```python
from build123d import *

# Parameters (mm, degrees)
SKETCH_1_W                  = 60
SKETCH_1_H                  = 100
EXTRUDE_1_DEPTH             = 2.9718
SKETCH_2_W                  = 2.9718
SKETCH_2_H                  = 40
CUT_EXTRUDE_1_DEPTH         = 10
SKETCH_4_W                  = 60
SKETCH_4_H                  = 30
EXTRUDE_2_DEPTH             = 2.9718
CUT_EXTRUDE_2_DEPTH         = 2.9718
PATTERN_LINEAR_1_COUNT      = 3
PATTERN_LINEAR_1_PITCH      = 8
SKETCH_5_R                  = 1
CUT_EXTRUDE_3_DEPTH         = 10
PATTERN_LINEAR_2_COUNT      = 3
PATTERN_LINEAR_2_PITCH      = 8
PATTERN_LINEAR_2_COUNT_DIR2 = 2
PATTERN_LINEAR_2_PITCH_DIR2 = 30
CUT_EXTRUDE_4_DEPTH         = 10
SKETCH_8_R                  = 1.4
CUT_EXTRUDE_5_DEPTH         = 10
PATTERN_LINEAR_3_COUNT      = 4
PATTERN_LINEAR_3_PITCH      = 70


with BuildPart() as part:
    # 草图1 → 凸台-拉伸1 (new body)
    with BuildSketch(Plane(origin=(0, 0, 0), x_dir=(1, 0, 0), z_dir=(0, 1, 0))):
        Rectangle(SKETCH_1_W, SKETCH_1_H)
    extrude(amount=EXTRUDE_1_DEPTH)

    # 草图2 → 切除-拉伸1 (cut)
    with BuildSketch(Plane(origin=(0, 0, 0), x_dir=(-1, 0, 0), z_dir=(0, -1, 0))):
        with Locations((28.5141, 0)):
            Rectangle(SKETCH_2_W, SKETCH_2_H)
    extrude(amount=-CUT_EXTRUDE_1_DEPTH, mode=Mode.SUBTRACT)

    # 草图4 → 凸台-拉伸2 (add)
    with BuildSketch(Plane.XZ):
        with Locations((0, -65)):
            Rectangle(SKETCH_4_W, SKETCH_4_H)
    extrude(amount=-EXTRUDE_2_DEPTH)

    # 草图3 → 切除-拉伸2 (cut)
    with BuildSketch(Plane(origin=(0, 0, 0), x_dir=(-1, 0, 0), z_dir=(0, -1, 0))):
        with BuildLine():
            Line((-12.5, 55.002516758), (-30, 55.002516758))
            Line((-30, 55.002516758), (-30, 53.002516758))
            Line((-30, 53.002516758), (-12.5, 53.002516758))
            ThreePointArc((-12.5, 53.002516758), (-11.5, 54.002516758), (-12.5, 55.002516758))
        make_face()
        with BuildLine():
            Line((30, 53.002516758), (30, 55.002516758))
            Line((30, 55.002516758), (12.5, 55.002516758))
            ThreePointArc((12.5, 55.002516758), (11.5, 54.002516758), (12.5, 53.002516758))
            Line((12.5, 53.002516758), (30, 53.002516758))
        make_face()
        with BuildLine():
            Line((8, 55.002516758), (-8, 55.002516758))
            ThreePointArc((-8, 55.002516758), (-9, 54.002516758), (-8, 53.002516758))
            Line((-8, 53.002516758), (8, 53.002516758))
            ThreePointArc((8, 53.002516758), (9, 54.002516758), (8, 55.002516758))
        make_face()
    cut_extrude_2 = extrude(amount=-CUT_EXTRUDE_2_DEPTH, mode=Mode.SUBTRACT)

    # 阵列(线性)1: 切除-拉伸2 ×3
    with Locations(*[(0, 0, -i * PATTERN_LINEAR_1_PITCH) for i in range(1, PATTERN_LINEAR_1_COUNT)]):
        add(cut_extrude_2, mode=Mode.SUBTRACT)

    # 草图5 → 切除-拉伸3 (cut)
    with BuildSketch(Plane.XZ):
        with BuildLine():
            Line((-5, -57.002516758), (-25, -57.002516758))
            ThreePointArc((-25, -57.002516758), (-24.292893219, -57.295409977), (-24, -58.002516758))
            ThreePointArc((-24, -58.002516758), (-24.292893219, -58.709623539), (-25, -59.002516758))
            Line((-25, -59.002516758), (-5, -59.002516758))
            ThreePointArc((-5, -59.002516758), (-6, -58.002516758), (-5, -57.002516758))
        make_face()
        with Locations((-25, -58.002516758)):
            Circle(SKETCH_5_R)
        with Locations((-5, -58.002516758)):
            Circle(SKETCH_5_R)
    cut_extrude_3 = extrude(amount=-CUT_EXTRUDE_3_DEPTH, mode=Mode.SUBTRACT)

    # 阵列(线性)2: Cut-Extrude 3 3 × 2
    with Locations(*[(j * PATTERN_LINEAR_2_PITCH_DIR2, 0, -i * PATTERN_LINEAR_2_PITCH) for i in range(PATTERN_LINEAR_2_COUNT) for j in range(PATTERN_LINEAR_2_COUNT_DIR2) if (i, j) != (0, 0)]):
        add(cut_extrude_3, mode=Mode.SUBTRACT)

    # 草图7 → 切除-拉伸4 (cut)
    with BuildSketch(Plane.XZ):
        Polygon((-30, 1.5), (-30, 0), (-15, 0), (-15, 1.5), (-19.5, 1.5), (-19.5, 4), (-22, 4), (-22, 1.5), align=None)
        Polygon((-30, 0), (-30, -1.5), (-22, -1.5), (-22, -4), (-19.5, -4), (-19.5, -1.5), (-15, -1.5), (-15, 0), align=None)
    extrude(amount=-CUT_EXTRUDE_4_DEPTH, mode=Mode.SUBTRACT)

    # 草图8 → 切除-拉伸5 (cut)
    with BuildSketch(Plane(origin=(0, 0, 0), x_dir=(-1, 0, 0), z_dir=(0, -1, 0))):
        with Locations((28.5, -35)):
            Circle(SKETCH_8_R)
    cut_extrude_5 = extrude(amount=-CUT_EXTRUDE_5_DEPTH, mode=Mode.SUBTRACT)

    # 阵列(线性)3: 切除-拉伸5 ×4
    with Locations(*[(0, 0, -i * PATTERN_LINEAR_3_PITCH) for i in range(1, PATTERN_LINEAR_3_COUNT)]):
        add(cut_extrude_5, mode=Mode.SUBTRACT)


solid = part.part
```
Input: part model. Units: mm. Frame: model coordinates. A direction names the side the tool comes from. Give positions to 0.01 mm unless a question says otherwise; leave off trailing zeros. Order: outer loops, then holes, each group sorted by start corner. A loop starts at its lowest first (then second) coordinate and runs counter-clockwise, first axis right, second up. Notation, with made-up numbers: M 12,40 L 21,40 A9 cw 21,54 Z; hole C -31,-30.5 d10. An arc over 180 degrees is marked long. One line per question, with ' | ' between items. Start each with the question number.
1. Section query D-D (y = 1.8). Count the separate pieces of the cut face and the enclosed holes in it, and give its area (3 significant figures).
2. Section query B-B (z = 35). Return the cut outline in (x, y), and give its area (3 significant figures).
3. Section query C-C (x = 23). Return the cut outline in (y, z), and give its area (3 significant figures).
4. First-contact query: pin 1 Ø0.8 at (y, z) = (1.5, 2.5) entering from -X. Flat tip, straight axial feed; report the tip coordinate or a pass-through.
5. Pull-direction query (Z, two-part tool) for faces 1 (the face through (-30, 1, -37)), 2 (the face through (0, 1, 50)), 3 (the face through (-28, 1, -20)), 4 (the face through (-15, 1, -75.003)); classes: released by +Z, released by -Z, zero draft, split by the parting line, or undercut.
6. Section query A-A (x = -28.5). Return the cut outline in (y, z).
7. Access query for faces 5 (the face through (21, 1, -61.003)), 6 (the face through (-17, 1, 1.5)), 7 (the face through (-30, 1, -66)), 8 (the face through (15, 1, -73.003)). Directions: +Z, -Z, +X, -X, +Y, -Y. A direction counts if a zero-diameter tool reaches every point of the face in a straight line with its end or side. Return the directions, or none.
8. Material intervals for probe 1 along Z at (x, y) = (10, 1.1); probe 2 along X at (y, z) = (2.1, -2.5); probe 3 along X at (y, z) = (0.3, 14.5), sorted ascending. Write a range as [from, to].
Here are the results:
1) separate pieces: 1 | enclosed holes: 11 | area: 7,040 mm²
2) outline: M -30,0 L -29.9,0 L -29.9,2.97 L -30,2.97 Z; M -27.1,0 L 30,0 L 30,2.97 L -27.1,2.97 Z | area: 170 mm²
3) outline: M 0,-80 L 2.97,-80 L 2.97,-75 L 0,-75 Z; M 0,-73 L 2.97,-73 L 2.97,-71 L 0,-71 Z; M 0,-69 L 2.97,-69 L 2.97,-67 L 0,-67 Z; M 0,-65 L 2.97,-65 L 2.97,-63 L 0,-63 Z; M 0,-61 L 2.97,-61 L 2.97,-59 L 0,-59 Z; M 0,-57 L 2.97,-57 L 2.97,-55 L 0,-55 Z; M 0,-53 L 2.97,-53 L 2.97,50 L 0,50 Z | area: 351 mm²
4) pin 1: x = -27.03
5) face 1: zero draft | face 2: released by +Z | face 3: undercut | face 4: undercut
6) outline: M 0,-80 L 2.97,-80 L 2.97,-71 L 0,-71 Z; M 0,-69 L 2.97,-69 L 2.97,-63 L 0,-63 Z; M 0,-61 L 2.97,-61 L 2.97,-55 L 0,-55 Z; M 0,-53 L 2.97,-53 L 2.97,-36.4 L 0,-36.4 Z; M 0,-33.6 L 2.97,-33.6 L 2.97,-20 L 0,-20 Z; M 0,20 L 2.97,20 L 2.97,33.6 L 0,33.6 Z; M 0,36.4 L 2.97,36.4 L 2.97,50 L 0,50 Z
7) face 5: +X, +Y, -Y | face 6: -X, +Y, -Y | face 7: +Z, -Z, -X, +Y, -Y | face 8: +Y, -Y
8) probe 1: [-80, -75], [-73, -67], [-65, -59], [-57, 50] | probe 2: [-27.03, -22], [-19.5, 30] | probe 3: [-27.03, 30]
